Geometry: see drawing. Coordinates: mm, zero at the bounding-box minimum. A direction names the side the tool comes from. Give positions to 0.01 mm unless a question says otherwise; leave off trailing zeros. Loops run counter-clockwise (first coordinate to the right, second up) from the corner with the lowest first, then second, coordinate; pieces in that order, holes last. Notation, with made-up numbers: (50, -22.75) - (60, -22.75) arc R11 cw to (60, -13.75) - close; hole circle Ø7 at (54, -26.5). An arc over 180 degrees is marked (long way). Use one line per item in the form item = value.
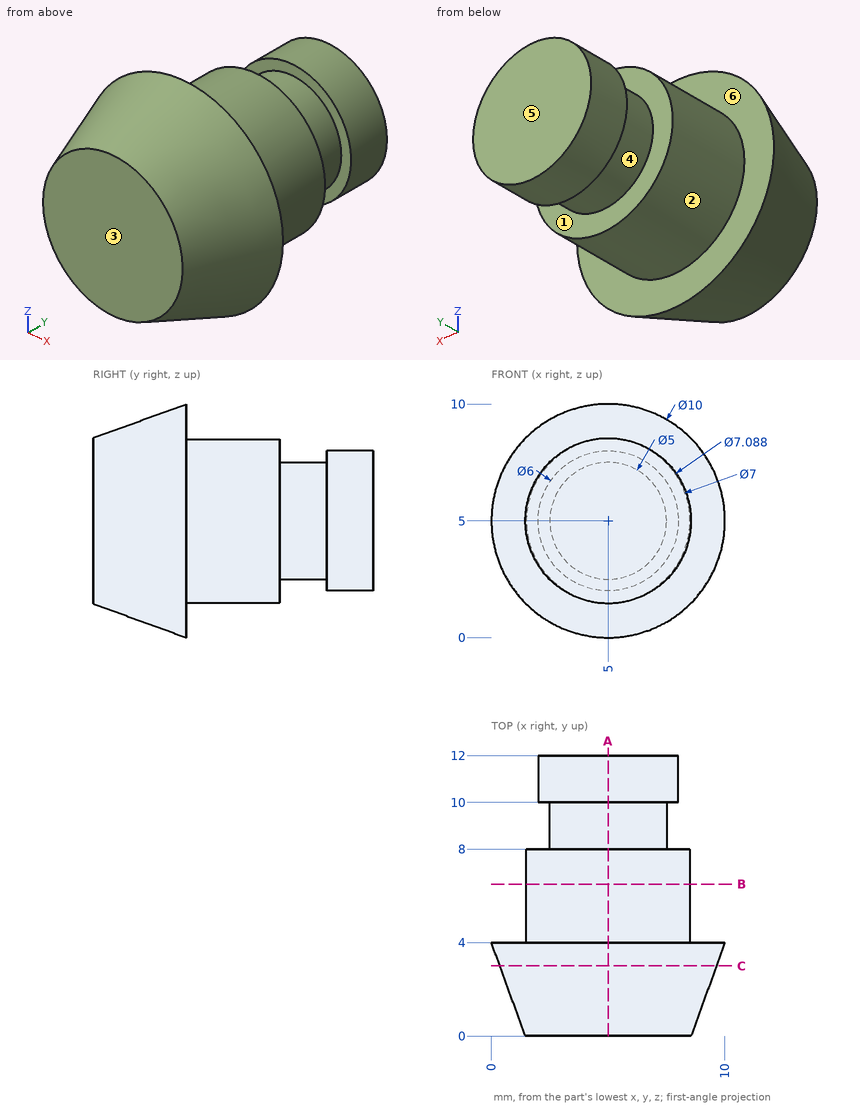
(1) Access query for the marked faces 4, 5 and 6. Directions: +Z, -Z, +X, -X, +Y, -Y. A direction counts if a zero-diameter tool reaches every point of the face in a straight line with its end or side. Return the directions, or none.
Solution:
face_4 = none
face_5 = +Z, -Z, +X, -X, +Y
face_6 = +Y
(2) Cut plane B-B (y = 6.5). Return the cut outline in (x, z), plus the area to 3 significant figures.
Solution:
outline = circle Ø7 at (5, 5)
area = 38.5 mm2
(3) Pin query (flat end, axial travel): P1, Ø1, axis at y = 9, z = 5.5, coming from the +X side; P2, Ø3, axis at y = 8.5, z = 2, coming from the +X side; P3, Ø1.5, axis at y = 10, z = 2, coming from the +X side (1 decimal). Return the tip coordinate at first contact, or that it passes through.
Solution:
P1 = 7.5
P2 = 8.12
P3 = 7
(4) Cut plane A-A (x = 5). Return the cut outline in (y, z), plus the area to 3 significant figures.
Solution:
outline = (0, 1.46) - (4, 0) - (4, 1.5) - (8, 1.5) - (8, 2.5) - (10, 2.5) - (10, 2) - (12, 2) - (12, 8) - (10, 8) - (10, 7.5) - (8, 7.5) - (8, 8.5) - (4, 8.5) - (4, 10) - (0, 8.54) - close
area = 84.2 mm2
(5) Cut plane C-C (y = 3). Return the cut outline in (x, z), plus the area to 3 significant figures.
Solution:
outline = circle Ø9.27 at (5, 5)
area = 67.5 mm2
(6) Material intervals for L1, parallel to Y at x = 7.25, z = 3.75; L2, parallel to Y at x = 4.25, z = 8.25; L3, parallel to Z at x = 1.5, y = 1.75, sorted ascending. Write a range as from..to.
Solution:
L1 = 0..8, 10..12
L2 = 0..8
L3 = 2.71..7.29
(7) Pull-direction query (Y, two-part tool) for the marked faces 1, 2 and 3; classes: released by +Y, released by -Y, zero draft, split by the parting line, or undercut.
Solution:
face_1 = undercut
face_2 = zero draft
face_3 = released by -Y
